```python
from build123d import *

# Parameters (mm, degrees)
F3_W     = 50.7285948843
F3_H     = 69.9163675308
F6_W     = 101.6
F6_H     = 101.6
F7_DEPTH = 25.4
F8_R     = 25.39999


# Not quite as in the source:
# - a fillet or chamfer is up to 0.001 mm smaller than in the source, because OpenCascade refuses the exact size


with BuildPart() as f4:
    # F1 (on offset) → F4 section 0
    with BuildSketch(Plane.YZ.offset(127)):
        with BuildLine():
            add(Edge.make_bspline(
                [(-11.8536790833, -25.3428127617), (16.5973998136, -117.2622232897), (89.6947664905, -44.2741583201), (162.7921331674, 28.7139066495), (61.2436875936, 47.6452522079), (-40.3047579802, 66.5765977664), (-11.8536790833, -25.3428127617)],
                knots=[0, 0, 0, 2.0943951024, 2.0943951024, 4.1887902048, 4.1887902048, 6.2831853072, 6.2831853072, 6.2831853072], degree=2, weights=[1, 0.5, 1, 0.5, 1, 0.5, 1]))
        make_face()
    # F3 (on offset) → F4 section 1
    with BuildSketch(Plane.XY.offset(254)):
        with Locations((-8.5154855624, -1.6246475279)):
            Rectangle(F3_W, F3_H)
    loft()


with BuildPart() as f7:
    # F6 (on offset) → F7 (new body)
    with BuildSketch(Plane.XY.offset(254)):
        with Locations((-0.4687514156, 6.5054772415)):
            Rectangle(F6_W, F6_H)
    extrude(amount=F7_DEPTH)

    # F8 (radius 25.4 in the source; OpenCascade refuses exactly that, so slightly less here)
    f8_edges = [f7.edges().sort_by_distance(p)[0] for p in [
        (50.331249, 6.505477, 279.4),
        (-0.468751, 57.305477, 279.4),
        (-51.268751, 6.505477, 279.4),
        (-0.468751, -44.294523, 279.4),
    ]]
    fillet(f8_edges, radius=F8_R)


solid = f7.part
```
Verification items for the finished model (mm, model axes). Round coordinates to 2 decimals unless told otherwise and drop trailing zeros. Order: outer loops, then holes, each group sorted by start corner. A loop starts at its lowest first (then second) coordinate and runs counter-clockwise, first axis right, second up. Notation, with made-up numbers: (44, 15) -> (72, 15) arc R21 ccw to (72, 22) -> close; hole circle Ø5 at (81, 46). An arc over 180 degrees is marked (long way). Put each result on its own line as item: value. Start each with the question number.
(1) Section check D-D (z = 260.5). Enter the section's corners in (x, y).
(2) Depth check by flat-ended pin: pin 1 Ø8 at (x, z) = (6, 257.5) entering from +Y; pin 2 Ø2 at (x, z) = (-40.5, 257.5) entering from +Y; pin 3 Ø5 at (y, z) = (-28, 273.5) entering from -X; pin 4 Ø1 at (x, y) = (-3.5, -20.5) entering from +Z. Enter the tip coordinate at first touch or a pass-through.
(3) Material ranges on line 1 along Z through (x, y) = (34, 42); line 2 along Z through (x, y) = (-8.5, 34.5); line 3 along X through (y, z) = (18, 267.5), recorded low to high.
(4) Section check C-C (z = 277.5). Enter the section's corners in (x, y), then the cut area to 3 significant figures.
Completed:
1. outline: (-50.42, -43.45) -> (49.49, -43.45) -> (49.49, 56.46) -> (-50.42, 56.46) -> close
2. pin 1: stops at y = 57.31
2. pin 2: stops at y = 57.18
2. pin 3: stops at x = -44.74
2. pin 4: stops at z = 279.38
3. line 1: z = 254 to 277.31
3. line 2: z = 254 to 279.27
3. line 3: x = -47.38 to 46.45
4. outline: (-35.51, -28.53) -> (34.57, -28.53) -> (34.57, 41.54) -> (-35.51, 41.54) -> close
4. area: 4,910 mm2
